The model under review builds one solid part; all positions refer to its coordinate system, in mm. A direction names the side the tool comes from. Give positions to 0.01 mm unless a question says otherwise; leave off trailing zeros. Order: outer loops, then holes, each group sorted by start corner. A loop starts at its lowest first (then second) coordinate and runs counter-clockwise, first axis right, second up. Notation, with made-up numbers: (83, 11) - (100, 11) arc R15 ccw to (100, 27) - close; hole circle Ø8 at (-37, -18.5). An arc over 180 degrees is marked (long way). Use CSV: the item, a comma, the result in double quotes.
```python
from build123d import *

# Parameters (mm, degrees)
F0_W     = 420
F0_H     = 460
F1_DEPTH = 15
F2_R     = 5
F3_DEPTH = 15
F4_W     = 402
F4_H     = 402
F5_DEPTH = 5.5


with BuildPart() as f1:
    # F0 (on Top) → F1 (new body)
    with BuildSketch(Plane.XY):
        with Locations((135.56531, 178.600564)):
            Rectangle(F0_W, F0_H)
    extrude(amount=F1_DEPTH)

    # F2 (on face) → F3 (cut)
    with BuildSketch(Plane.XY.offset(15)):
        with Locations((245.56531, -41.399436)):
            Circle(F2_R)
        with Locations((-44.43469, -41.399436)):
            Circle(F2_R)
        with Locations((100.56531, -41.399436)):
            Circle(F2_R)
        with Locations((245.56531, 398.600564)):
            Circle(F2_R)
        with Locations((100.56531, 398.600564)):
            Circle(F2_R)
        with Locations((-44.43469, 398.600564)):
            Circle(F2_R)
    extrude(amount=-F3_DEPTH, mode=Mode.SUBTRACT)

    # F4 (on face) → F5 (cut)
    with BuildSketch(Plane(origin=(0, 0, 0), x_dir=(1, 0, 0), z_dir=(0, 0, -1))):
        with Locations((135.56531, -178.600564)):
            Rectangle(F4_W, F4_H)
    extrude(amount=-F5_DEPTH, mode=Mode.SUBTRACT)


solid = f1.part
```
Item 1: Take a section at C-C, the plane z = 2.75. Give the boundary of the cut face in (x, y), and give its area (3 significant figures).
Results list:
outline,"(-74.43, -51.4) - (345.57, -51.4) - (345.57, 408.6) - (-74.43, 408.6) - close; hole (-65.43, -22.4) - (336.57, -22.4) - (336.57, 379.6) - (-65.43, 379.6) - close; hole circle Ø10 at (-44.43, -41.4); hole circle Ø10 at (-44.43, 398.6); hole circle Ø10 at (100.57, -41.4); hole circle Ø10 at (100.57, 398.6); hole circle Ø10 at (245.57, -41.4); hole circle Ø10 at (245.57, 398.6)"
area,"31,100 mm2"
Item 2: Take a section at B-B, the plane y = -13. Give the boundary of the cut face in (x, z).
Results list:
outline,"(-74.43, 0) - (-65.43, 0) - (-65.43, 5.5) - (336.57, 5.5) - (336.57, 0) - (345.57, 0) - (345.57, 15) - (-74.43, 15) - close"
Item 3: Tool access review of faces 4 (the face through (133, 176, 5.5)), 5 (the face through (247.873, 394.165, 7.605)): name each direction out of +Z, -Z, +X, -X, +Y, -Y from which nothing blocks a thin tool from reaching the whole face with its end or side.
Results list:
face 4,"-Z"
face 5,"+Z, -Z"
Item 4: Mouldability with a two-part tool opening along X and no side actions: class faces 1 (the face through (99.914, -36.442, 7.605)), 2 (the face through (133, 408.601, 7)), 3 (the face through (-74.435, 175, 7)) as pulls with the +X half, pulls with the -X half, needs draft (parallel to the pull), parting line crosses it, or undercut.
Results list:
face 1,"undercut"
face 2,"needs draft"
face 3,"pulls with the -X half"
Item 5: Take a section at A-A, the plane x = 195. Give the boundary of the cut face in (y, z), and give its area (3 significant figures).
Results list:
outline,"(-51.4, 0) - (-22.4, 0) - (-22.4, 5.5) - (379.6, 5.5) - (379.6, 0) - (408.6, 0) - (408.6, 15) - (-51.4, 15) - close"
area,"4,690 mm2"
Item 6: Wall thickness on L1, parallel to Y at x = 90, z = 0.5; L2, parallel to X at y = 86, z = 3.25; L3, parallel to Z at x = 39, y = 337: over which ranges is each line inside the solid? List them lowest first.
Results list:
L1,"y = -51.4 to -22.4, 379.6 to 408.6"
L2,"x = -74.43 to -65.43, 336.57 to 345.57"
L3,"z = 5.5 to 15"
Item 7: Clearance check with a flat-ended pin moving along its axis: pin 1 (12 mm diameter, centred on x = 216.5, y = 81, fed in from -Z). State where the tip first meets the part, or that it passes through.
Results list:
pin 1,"stops at z = 5.5"
